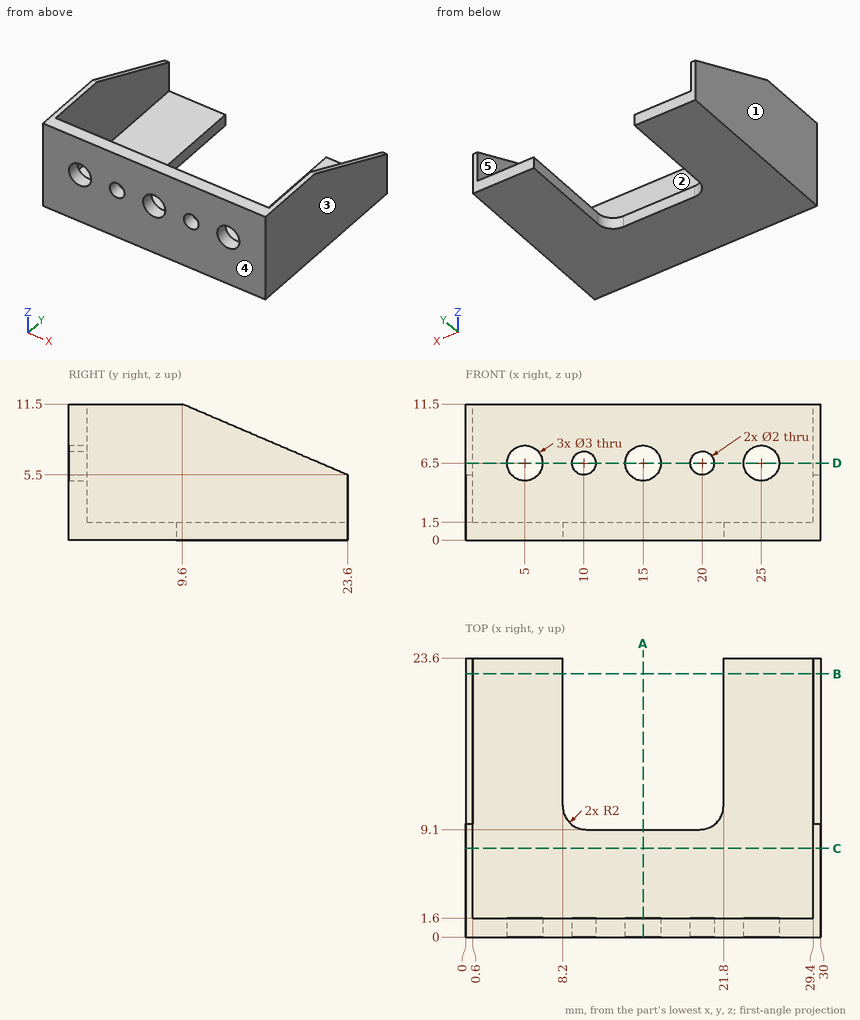
Design review of the part shown in the three views and the two pictorial views. Dimensions are in mm from the part's minimum x, y and z. A direction names the side the tool comes from. Give positions to 0.01 mm unless a question says otherwise; leave off trailing zeros. Write each loop counter-clockwise with the first axis right and the second up, starting at its lowest first coordinate (ties: lowest second). Pieces come first, ordered by that corner, then holes.
Item 1: The part is to be moulded in two halves that separate along X. For the marked faces 3, 4 and 5, say which applies: +X half, -X half, draft (parallel to the pull), parting line (faces both ways), or undercut.
Item 2: Machinability: for the marked faces 1 and 2, which of the approach directions +Z, -Z, +X, -X, +Y, -Y give a long, thin tool a straight path to every point of the face, cutting with its end or side? Answer none if there is none.
Item 3: Take a section at B-B (y = 22.25). Give the boundary of the cut face in (x, z).
Item 4: Take a section at A-A (x = 15). Give the boundary of the cut face in (y, z), and give its area (4 significant figures).
Item 5: Take a section at D-D (z = 6.5). Give the boundary of the cut face in (x, y).
Item 6: Insertion check: P1, Ø4, axis at x = 22, y = 20.5, coming from the +Z side; P2, Ø1.6, axis at x = 13, z = 0.5, coming from the +Y side; P3, Ø5, axis at x = 15, z = 6.5, coming from the +Y side. Each pin has a flat end and moves straight along its axis. Give the tip position at first contact, or say it passes through.
Item 7: Take a section at C-C (y = 7.5). Give the boundary of the cut face in (x, z), and give its area (3 significant figures).
Item 8: Wall thickness on probe 1 along X at (y, z) = (0.7, 6.5); probe 2 along X at (y, z) = (20.5, 4.25); probe 3 along Z at (x, y) = (5, 0.7): over which ranges is each line inside the solid? List them lowest first.
Established:
1. face 3: +X half
1. face 4: draft
1. face 5: undercut
2. face 1: +Z, -Z, -X, +Y, -Y
2. face 2: +Z, +Y
3. outline: (0, 0) - (8.2, 0) - (8.2, 1.5) - (0.6, 1.5) - (0.6, 6.08) - (0, 6.08) - close; (21.8, 0) - (30, 0) - (30, 6.08) - (29.4, 6.08) - (29.4, 1.5) - (21.8, 1.5) - close
4. outline: (0, 0) - (9.1, 0) - (9.1, 1.5) - (1.6, 1.5) - (1.6, 5) - (0, 5) - close; (0, 8) - (1.6, 8) - (1.6, 11.5) - (0, 11.5) - close
4. area: 24.85 mm2
5. outline: (0, 0) - (3.5, 0) - (3.5, 1.6) - (0.6, 1.6) - (0.6, 21.27) - (0, 21.27) - close; (6.5, 0) - (9, 0) - (9, 1.6) - (6.5, 1.6) - close; (11, 0) - (13.5, 0) - (13.5, 1.6) - (11, 1.6) - close; (16.5, 0) - (19, 0) - (19, 1.6) - (16.5, 1.6) - close; (21, 0) - (23.5, 0) - (23.5, 1.6) - (21, 1.6) - close; (26.5, 0) - (30, 0) - (30, 21.27) - (29.4, 21.27) - (29.4, 1.6) - (26.5, 1.6) - close
6. P1: stops at z = 1.5
6. P2: stops at y = 9.1
6. P3: stops at y = 1.6
7. outline: (0, 0) - (30, 0) - (30, 11.5) - (29.4, 11.5) - (29.4, 1.5) - (0.6, 1.5) - (0.6, 11.5) - (0, 11.5) - close
7. area: 57.0 mm2
8. probe 1: x = 0 to 3.5, 6.5 to 9, 11 to 13.5, 16.5 to 19, 21 to 23.5, 26.5 to 30
8. probe 2: x = 0 to 0.6, 29.4 to 30
8. probe 3: z = 0 to 5, 8 to 11.5
